```python
from build123d import *

# Parameters (mm, degrees)
RESSALTO_EXTRUS_O1_DEPTH = 5
ESBO_O2_R                = 2.25
CORTE_EXTRUS_O1_DEPTH    = 117.030017788
FILETE1_R                = 15


with BuildPart() as part:
    # Esboço1 → Ressalto-extrusão1 (new body)
    with BuildSketch(Plane.XY):
        with BuildLine():
            Line((-18.15, 0), (-18.15, 37.6))
            add(Edge.make_bspline(
                [(-18.15, 37.6), (-15.473970767, 49.184313893), (-10.375, 59.65)],
                knots=[0, 0, 0, 0.611079356, 0.611079356, 0.611079356], degree=2))
            add(Edge.make_bspline(
                [(-10.375, 59.65), (-10.182305069, 61.008012224), (-10.375, 62.25)],
                knots=[0, 0, 0, 0.268489531, 0.268489531, 0.268489531], degree=2))
            add(Edge.make_bspline(
                [(-10.375, 62.25), (-17.376864496, 67.749205026), (-20.75, 75.25)],
                knots=[0, 0, 0, 0.738516148, 0.738516148, 0.738516148], degree=2))
            Line((-20.75, 75.25), (-20.75, 114.05))
            Line((-20.75, 114.05), (15.6, 114.05))
            Line((15.6, 114.05), (15.6, 75.25))
            add(Edge.make_bspline(
                [(10.375, 62.25), (14.919065783, 68.376354775), (15.6, 75.25)],
                knots=[0, 0, 0, 0.739355324, 0.739355324, 0.739355324], degree=2))
            add(Edge.make_bspline(
                [(10.375, 59.65), (10.182305069, 61.008012224), (10.375, 62.25)],
                knots=[0, 0, 0, 0.268489531, 0.268489531, 0.268489531], degree=2))
            add(Edge.make_bspline(
                [(18.15, 37.6), (15.473970767, 49.184313893), (10.375, 59.65)],
                knots=[0, 0, 0, 0.611079356, 0.611079356, 0.611079356], degree=2))
            Line((18.15, 37.6), (18.15, 0))
            ThreePointArc((18.15, 0), (0, -18.15), (-18.15, 0))
        make_face()
    extrude(amount=RESSALTO_EXTRUS_O1_DEPTH)

    # Esboço2 → Corte-extrusão1 (cut, through all)
    with BuildSketch(Plane.XY.offset(5)):
        with Locations((-0.31, -6.15)):
            Circle(ESBO_O2_R)
        with Locations((-2.575, 106.05)):
            Circle(ESBO_O2_R)
    extrude(amount=-CORTE_EXTRUS_O1_DEPTH, mode=Mode.SUBTRACT)

    # Filete1
    filete1_edges = [part.edges().sort_by_distance(p)[0] for p in [
        (-20.75, 114.05, 2.5),
        (15.6, 114.05, 2.5),
    ]]
    fillet(filete1_edges, radius=FILETE1_R)


solid = part.part
```
Check sheet for the modelled part. Datum: model origin and axes. Units: mm. A direction names the side the tool comes from. Round coordinates to 2 decimals unless told otherwise and drop trailing zeros. Loops run counter-clockwise (first coordinate to the right, second up) from the corner with the lowest first, then second, coordinate; pieces in that order, holes last. Notation, with made-up numbers: M -19.5,31.5 L 35.5,31.5 A19 cw 35.5,37.5 Z; hole C 19.25,31 d6. An arc over 180 degrees is marked long. Answer as a JSON object with one key per item and string values.
1. Gauge pin test, flat ends, axial feed: P1, Ø3.5, axis at x = -0.31, y = -6.15, coming from the +Z side; P2, Ø1.5, axis at y = 35, z = 4.5, coming from the -X side. Record the tip position at first contact, or that the pin passes through.
Reply:
{"P1": "passes through", "P2": "stops at x = -18.15"}
2. Section check A-A (y = 106.05). Record the boundary of the cut face in (x, z) (1 decimal), plus the area to 3 significant figures.
Reply:
{"outline": "M -19,0 L -4.8,0 L -4.8,5 L -19,5 Z; M -0.3,0 L 13.9,0 L 13.9,5 L -0.3,5 Z", "area": "142 mm²"}
3. Scan lines: line 1 (X direction, y = -6, z = 2.9) (3 decimals); line 2 (Y direction, x = 11, z = 2.4); line 3 (X direction, y = 81.5, z = 4.5). Record each from-to range of solid material in increasing order.
Reply:
{"line 1": "x = -17.13 to -2.555, 1.935 to 17.13", "line 2": "y = -14.44 to 58.34, 63.12 to 109.86", "line 3": "x = -20.75 to 15.6"}
4. Section check C-C (y = 3). Record the boundary of the cut face in (x, z), plus the area to 4 significant figures.
Reply:
{"outline": "M -18.15,0 L 18.15,0 L 18.15,5 L -18.15,5 Z", "area": "181.5 mm²"}
5. Mould release check, pull along X, two halves, no side actions. Record for faces 1 (the flat face through (-1, 49, 0)), 2 (the cylindrical face through (1.836, -5.474, 2.535)), 3 (the flat face through (18.15, 19, 2)): pulls with the +X half, pulls with the -X half, needs draft (parallel to the pull), parting line crosses it, or undercut.
Reply:
{"face 1": "needs draft", "face 2": "undercut", "face 3": "pulls with the +X half"}
6. Section check D-D (x = 8). Record the boundary of the cut face in (y, z), plus the area to 3 significant figures.
Reply:
{"outline": "M -16.29,0 L 112.1,0 L 112.1,5 L -16.29,5 Z", "area": "642 mm²"}
7. Section check B-B (z = 3.2). State how many separate pieces and enclosed holes the cut face has, plus the area to 3 significant figures.
Reply:
{"separate pieces": "1", "enclosed holes": "2", "area": "4,260 mm²"}
8. Access from +Z, -Z, +X, -X, +Y, -Y to the whole of each face (thin tool, end or side, straight path). Record for faces 4 (the cylindrical face through (-16, 110, 3)), 5 (the flat face through (-18.15, 19, 2)), 6 (the flat face through (15.6, 87, 2)).
Reply:
{"face 4": "+Z, -Z, -X, +Y", "face 5": "+Z, -Z, -X, -Y", "face 6": "+Z, -Z, +X, +Y"}
